For this review, take the finished solid that the model builds, in its own axes (mm). A direction names the side the tool comes from. Give positions to 0.01 mm unless a question says otherwise; leave off trailing zeros. Order: outer loops, then holes, each group sorted by start corner. A loop starts at its lowest first (then second) coordinate and runs counter-clockwise, first axis right, second up.
from build123d import *

# Parameters (mm, degrees)
SKETCH_W   = 276
SKETCH_H   = 41
SKETCH_W_2 = 11
SKETCH_H_2 = 11
PAD_DEPTH  = 11
FILLET_R   = 3


with BuildPart() as part:
    # Sketch → Pad (new body)
    with BuildSketch(Plane.XY):
        Rectangle(SKETCH_W, SKETCH_H)
        with Locations((-102.5, 0)):
            Rectangle(SKETCH_W_2, SKETCH_H_2, mode=Mode.SUBTRACT)
        with Locations((-61.5, 0)):
            Rectangle(SKETCH_W_2, SKETCH_H_2, mode=Mode.SUBTRACT)
        with Locations((-20.5, 0)):
            Rectangle(SKETCH_W_2, SKETCH_H_2, mode=Mode.SUBTRACT)
        with Locations((20.5, 0)):
            Rectangle(SKETCH_W_2, SKETCH_H_2, mode=Mode.SUBTRACT)
        with Locations((61.5, 0)):
            Rectangle(SKETCH_W_2, SKETCH_H_2, mode=Mode.SUBTRACT)
        with Locations((102.5, 0)):
            Rectangle(SKETCH_W_2, SKETCH_H_2, mode=Mode.SUBTRACT)
    extrude(amount=PAD_DEPTH)

    # Fillet
    fillet_edges = [part.edges().sort_by_distance(p)[0] for p in [
        (-138, 0, 11),
        (0, -20.5, 11),
        (138, 0, 11),
        (0, 20.5, 11),
        (97, 0, 11),
        (102.5, -5.5, 11),
        (108, 0, 11),
        (102.5, 5.5, 11),
        (56, 0, 11),
        (61.5, -5.5, 11),
        (67, 0, 11),
        (61.5, 5.5, 11),
        (15, 0, 11),
        (20.5, -5.5, 11),
        (26, 0, 11),
        (20.5, 5.5, 11),
        (-26, 0, 11),
        (-20.5, -5.5, 11),
        (-15, 0, 11),
        (-20.5, 5.5, 11),
        (-67, 0, 11),
        (-61.5, -5.5, 11),
        (-56, 0, 11),
        (-61.5, 5.5, 11),
        (-108, 0, 11),
        (-102.5, -5.5, 11),
        (-97, 0, 11),
        (-102.5, 5.5, 11),
    ]]
    fillet(fillet_edges, radius=FILLET_R)


solid = part.part
1) Tool access review of faces 4 (the face through (26, 0, 4)), 5 (the face through (-2, -20.5, 4)): name each direction out of +Z, -Z, +X, -X, +Y, -Y from which nothing blocks a thin tool from reaching the whole face with its end or side.
Answer sheet:
face 4: +Z, -Z
face 5: +Z, -Z, +X, -X, -Y
2) Clearance check with a flat-ended pin moving along its axis: pin 1 (1.5 mm diameter, centred on x = 15, z = 9.5, fed in from -Y). State where the tip first meets the part, or that it passes through.
Answer sheet:
pin 1: stops at y = -20.4
3) We need section A-A on x = -101. Give the boundary of the cut face in (y, z), then the cut area to 3 significant figures.
Answer sheet:
outline: (-20.5, 0) - (-5.5, 0) - (-5.5, 8) arc R3 ccw to (-8.5, 11) - (-17.5, 11) arc R3 ccw to (-20.5, 8) - close; (5.5, 0) - (20.5, 0) - (20.5, 8) arc R3 ccw to (17.5, 11) - (8.5, 11) arc R3 ccw to (5.5, 8) - close
area: 322 mm2
4) We need section B-B on z = 2. Give the boundary of the cut face in (x, y).
Answer sheet:
outline: (-138, -20.5) - (138, -20.5) - (138, 20.5) - (-138, 20.5) - close; hole (-108, -5.5) - (-97, -5.5) - (-97, 5.5) - (-108, 5.5) - close; hole (-67, -5.5) - (-56, -5.5) - (-56, 5.5) - (-67, 5.5) - close; hole (-26, -5.5) - (-15, -5.5) - (-15, 5.5) - (-26, 5.5) - close; hole (15, -5.5) - (26, -5.5) - (26, 5.5) - (15, 5.5) - close; hole (56, -5.5) - (67, -5.5) - (67, 5.5) - (56, 5.5) - close; hole (97, -5.5) - (108, -5.5) - (108, 5.5) - (97, 5.5) - close
5) We need section C-C on y = -3. Count the separate pieces of the cut face and the enclosed holes in it, then the cut area to 3 significant figures.
Answer sheet:
separate pieces: 7
enclosed holes: 0
area: 2,280 mm2
6) Draft analysis for pull direction X (two halves, no side actions). For faces 1 (the face through (-138, 0, 4)), 2 (the face through (-2, 20.5, 4)), 3 (the face through (-15, 0, 4)), state which applies: +X half, -X half, draft (parallel to the pull), parting line (faces both ways), or undercut.
Answer sheet:
face 1: -X half
face 2: draft
face 3: undercut
7) To check wall thickness, follow line 1 (Y direction, x = 103, z = 8); line 2 (Y direction, x = 20, z = 10.25); line 3 (Y direction, x = -76, z = 9). State the ranges of each line that lie inside material, in increasing order.
Answer sheet:
line 1: y = -20.5 to -5.5, 5.5 to 20.5
line 2: y = -19.48 to -6.52, 6.52 to 19.48
line 3: y = -20.33 to 20.33
